Read the model definition and answer for the solid it produces. Units are mm, in the model's axes. A direction names the side the tool comes from. Coordinates: 2 decimals unless noted, no trailing zeros. Loops run counter-clockwise (first coordinate to the right, second up) from the corner with the lowest first, then second, coordinate; pieces in that order, holes last.
from build123d import *

# Parameters (mm, degrees)
CROQUIS1_R              = 55
SALIENTE_EXTRUIR1_DEPTH = 5
CROQUIS2_R              = 49
SALIENTE_EXTRUIR2_DEPTH = 30
CROQUIS3_R              = 2
CROQUIS4_R              = 44
CORTAR_EXTRUIR1_DEPTH   = 31


with BuildPart() as part:
    # Croquis1 → Saliente-Extruir1 (new body)
    with BuildSketch(Plane.XY):
        Circle(CROQUIS1_R)
    extrude(amount=SALIENTE_EXTRUIR1_DEPTH)

    # Croquis2 → Saliente-Extruir2 (add)
    with BuildSketch(Plane.XY.offset(5)):
        Circle(CROQUIS2_R)
    extrude(amount=SALIENTE_EXTRUIR2_DEPTH)

    # Croquis3 → Cortar-Revolución1 (revolve, cut)
    with BuildSketch(Plane(origin=(0, 0, 0), x_dir=(1, 0, 0), z_dir=(0, 1, 0)), mode=Mode.PRIVATE) as cortar_revoluci_n1_sk:
        with Locations((-49, -15)):
            Circle(CROQUIS3_R)
        with Locations((-49, -27)):
            Circle(CROQUIS3_R)
    revolve(cortar_revoluci_n1_sk.sketch.rotate(Axis((0, 0, 36.878025431), (0, 0, -1)), 180), axis=Axis((0, 0, 36.878025431), (0, 0, -1)), mode=Mode.SUBTRACT)

    # Croquis4 → Cortar-Extruir1 (cut)
    with BuildSketch(Plane.XY.offset(35)):
        Circle(CROQUIS4_R)
    extrude(amount=-CORTAR_EXTRUIR1_DEPTH, mode=Mode.SUBTRACT)


solid = part.part
Q1. A cutting plane is placed at B-B (y = 0). Give the vertices of the cut face in (x, z), then the cut area to 3 significant figures.
Findings below:
outline: (-55, 0) - (55, 0) - (55, 5) - (49, 5) - (49, 13) arc R2 cw to (49, 17) - (49, 25) arc R2 cw to (49, 29) - (49, 35) - (44, 35) - (44, 4) - (-44, 4) - (-44, 35) - (-49, 35) - (-49, 29) arc R2 cw to (-49, 25) - (-49, 17) arc R2 cw to (-49, 13) - (-49, 5) - (-55, 5) - close
area: 737 mm2
Q2. Which of the six approach directions +Z, -Z, +X, -X, +Y, -Y give full straight-line access (tool end or side, diameter ignored) to faces 1 (the face through (-11.923, -53.692, 2.465)), 2 (the face through (-9.538, -42.954, 19.717))?
Findings below:
face 1: +Z, -Z
face 2: +Z
Q3. Determine the mould class of faces 3 (the face through (-40.2, 18.4, 35)), 4 (the face through (26.34, 41.32, 31.96)), 5 (the face through (-1, 1, 4)) for opening direction X: +X half, -X half, draft (parallel to the pull), parting line (faces both ways), or undercut.
Findings below:
face 3: draft
face 4: parting line
face 5: undercut
Q4. Flat-ended cylindrical pins translate along their axes: pin 1 Ø1.5 at (y, z) = (15.5, 7) entering from -X; pin 2 Ø3 at (x, z) = (-43, 17.5) entering from -Y; pin 3 Ø8 at (x, y) = (20.5, 18.5) entering from +Z. Find the tip coordinate at first contact, or state that the pin passes through.
Findings below:
pin 1: stops at x = -46.73
pin 2: stops at y = -26.05
pin 3: stops at z = 4
Q5. A cutting plane is placed at A-A (z = 8). Give the vertices of the cut face in (x, y), then the cut area to 3 significant figures.
Findings below:
outline: circle Ø98 at (0, 0); hole circle Ø88 at (0, 0)
area: 1,460 mm2
Q6. Straight lines are drawn through the part: probe 1 along Z at (x, y) = (-4, 38); probe 2 along X at (y, z) = (-26.5, 6); probe 3 along X at (y, z) = (39, 21). For each, find the intervals that lie inside material, in ascending order.
Findings below:
probe 1: z = 0 to 4
probe 2: x = -41.22 to -35.12, 35.12 to 41.22
probe 3: x = -29.66 to -20.37, 20.37 to 29.66
